Verification items for this drawing (mm, ordinates from the low corner). A direction names the side the tool comes from. Round coordinates to 2 decimals unless told otherwise and drop trailing zeros. Loops run counter-clockwise (first coordinate to the right, second up) from the corner with the lowest first, then second, coordinate; pieces in that order, holes last. Notation, with made-up numbers: (-21, 3.5) - (14, 3.5) arc R32 cw to (14, 29.5) - close; hole circle Ø2 at (76.25, -22). An arc over 180 degrees is marked (long way). Use a Markdown table: item, result. Add a question column.
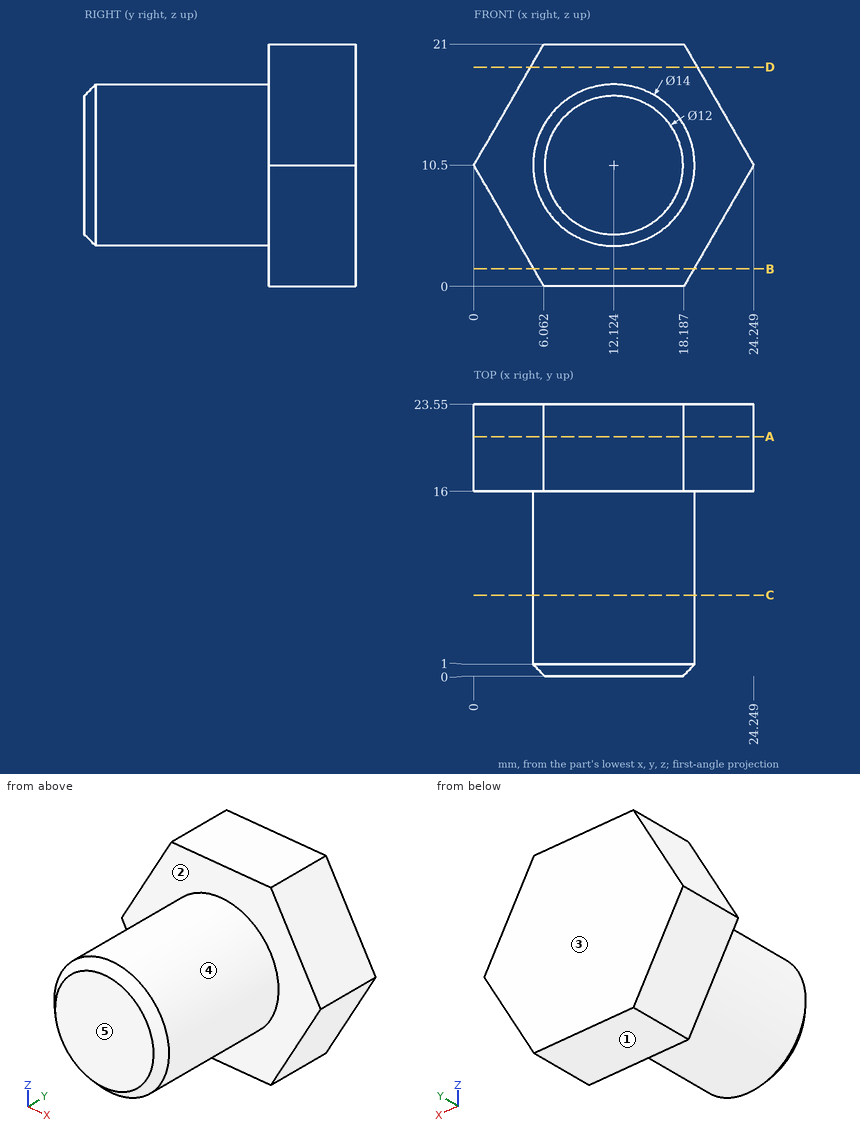
Q1. Section check C-C on y = 7. Record the cut outline in (x, z) (1 decimal), plus the area to 3 significant figures.
Q2. Release check for a two-part mould opening along Y. For the marked faces 3, 4 and 5 record: +Y half, -Y half, draft (parallel to the pull), parting line (faces both ways), or undercut.
Q3. Set-up check for the marked faces 1 and 2: record each of +Z, -Z, +X, -X, +Y, -Y from which the full face is reachable in a straight line by a thin tool's end or side.
Q4. Thickness scan on line 1 along Y through (x, z) = (9, 2.5); line 2 along X through (y, z) = (4.5, 10.5) (1 decimal); line 3 along X through (y, z) = (16.75, 5.5) (1 decimal). Record the ranges inside material, lowest first.
Q5. Section check A-A on y = 20.75. Record the cut outline in (x, z).
Q6. Section check D-D on z = 19. Record the cut outline in (x, y), plus the area to 3 significant figures.
Q7. Section check B-B on z = 1.5. Record the cut outline in (x, y), plus the area to 3 significant figures.
Q8. Go/stop test with flat-tipped pins: pin 1 Ø8 at (x, y) = (2.5, 5) entering from +Z (1 decimal); pin 2 Ø6 at (x, y) = (21.5, 14) entering from +Z (1 decimal); pin 3 Ø4 at (x, z) = (16.5, 2.5) entering from -Y. Record where each tip stops, or that it passes through.
Determined:
| question | item | result |
|---|---|---|
| 1 | outline | circle Ø14 at (12.1, 10.5) |
| 1 | area | 154 mm² |
| 2 | face 3 | +Y half |
| 2 | face 4 | draft |
| 2 | face 5 | -Y half |
| 3 | face 1 | -Z, +X, -X, +Y, -Y |
| 3 | face 2 | -Y |
| 4 | line 1 | y = 16 to 23.55 |
| 4 | line 2 | x = 5.1 to 19.1 |
| 4 | line 3 | x = 2.9 to 21.4 |
| 5 | outline | (0, 10.5) - (6.06, 0) - (18.19, 0) - (24.25, 10.5) - (18.19, 21) - (6.06, 21) - close |
| 6 | outline | (4.91, 16) - (19.34, 16) - (19.34, 23.55) - (4.91, 23.55) - close |
| 6 | area | 109 mm² |
| 7 | outline | (5.2, 16) - (19.05, 16) - (19.05, 23.55) - (5.2, 23.55) - close |
| 7 | area | 105 mm² |
| 8 | pin 1 | stops at z = 14.7 |
| 8 | pin 2 | stops at z = 19.1 |
| 8 | pin 3 | stops at y = 16 |
